from build123d import *

# Parameters (mm, degrees)
BOSS_EXTRUDE1_DEPTH       = 17.5
BOSS_EXTRUDE2_DEPTH       = 12.5
BOSS_EXTRUDE3_DEPTH       = 8
FILLET1_RADIUS            = 8
FILLET1_LENGTH            = 5
FILLET2_RADIUS            = 8
FILLET2_LENGTH            = 5
F_6_0MM_DOWEL_HOLE1_D     = 6
F_6_0MM_DOWEL_HOLE1_DEPTH = 21.06015
F_6_0MM_DOWEL_HOLE2_D     = 6
F_6_0MM_DOWEL_HOLE2_DEPTH = 12


with BuildPart() as part:
    # Sketch1 → Boss-Extrude1 (new, symmetric)
    with BuildSketch(Plane(origin=(0, 0, 0), x_dir=(0, 0, -1), z_dir=(1, 0, 0))):
        with BuildLine():
            Line((-7.858116823, -1.5), (-12.409673646, -1.5))
            ThreePointArc((-12.409673646, -1.5), (-8.291561976, -9.354143467), (0, -12.5))
            ThreePointArc((0, -12.5), (8.485281374, -16.014718626), (12, -24.5))
            Line((12, -24.5), (12, -33))
            Line((12, -33), (33, -33))
            Line((33, -33), (33, -3))
            Line((33, -3), (12.1346611, -3))
            ThreePointArc((12.1346611, -3), (2.254197856, 12.295063726), (-12.409673646, 1.5))
            Line((-12.409673646, 1.5), (-7.858116823, 1.5))
            ThreePointArc((-7.858116823, 1.5), (8, 0), (-7.858116823, -1.5))
        make_face()
    extrude(amount=BOSS_EXTRUDE1_DEPTH, both=True)

    # Sketch1<3> → Boss-Extrude2 (add, symmetric)
    with BuildSketch(Plane(origin=(0, 0, 0), x_dir=(0, 0, -1), z_dir=(1, 0, 0))):
        with BuildLine():
            ThreePointArc((-6, 10.9658561), (0, 12.5), (6, 10.9658561))
            Line((6, 10.9658561), (6, 25))
            Line((6, 25), (-6, 25))
            Line((-6, 25), (-6, 10.9658561))
        make_face()
    extrude(amount=BOSS_EXTRUDE2_DEPTH, both=True)

    # Sketch1<4> → Boss-Extrude3 (add, symmetric)
    with BuildSketch(Plane(origin=(0, 0, 0), x_dir=(0, 0, -1), z_dir=(1, 0, 0))):
        with BuildLine():
            ThreePointArc((-12.409673646, 1.5), (-11.810991842, 4.092734013), (-10.677078252, 6.5))
            Line((-10.677078252, 6.5), (-25, 6.5))
            Line((-25, 6.5), (-25, 1.5))
            Line((-25, 1.5), (-12.409673646, 1.5))
        make_face()
        with BuildLine():
            Line((-25, -6.5), (-10.677078252, -6.5))
            ThreePointArc((-10.677078252, -6.5), (-11.810991842, -4.092734013), (-12.409673646, -1.5))
            Line((-12.409673646, -1.5), (-25, -1.5))
            Line((-25, -1.5), (-25, -6.5))
        make_face()
    extrude(amount=BOSS_EXTRUDE3_DEPTH, both=True)

    # Fillet1: full round fillet: the end face becomes a half cylinder, R = half its width
    fillet1_face = Plane((0, 4, 25), x_dir=(0, 1, 0), z_dir=(0, 0, 1))  # on the end face: x along it, z out of the body
    fillet1_slab = fillet1_face.offset(-FILLET1_RADIUS / 2) * Box(FILLET1_LENGTH, 2 * FILLET1_RADIUS, FILLET1_RADIUS, mode=Mode.PRIVATE)  # the body's end, R deep
    fillet1_round = Plane((0, 4, 17), x_dir=(0, 0, 1), z_dir=(0, 1, 0)) * Cylinder(FILLET1_RADIUS, FILLET1_LENGTH, mode=Mode.PRIVATE)  # its axis R under the face
    add(fillet1_slab - fillet1_round, mode=Mode.SUBTRACT)

    # Fillet2: full round fillet: the end face becomes a half cylinder, R = half its width
    fillet2_face = Plane((0, -4, 25), x_dir=(0, -1, 0), z_dir=(0, 0, 1))  # on the end face: x along it, z out of the body
    fillet2_slab = fillet2_face.offset(-FILLET2_RADIUS / 2) * Box(FILLET2_LENGTH, 2 * FILLET2_RADIUS, FILLET2_RADIUS, mode=Mode.PRIVATE)  # the body's end, R deep
    fillet2_round = Plane((0, -4, 17), x_dir=(0, 0, 1), z_dir=(0, -1, 0)) * Cylinder(FILLET2_RADIUS, FILLET2_LENGTH, mode=Mode.PRIVATE)  # its axis R under the face
    add(fillet2_slab - fillet2_round, mode=Mode.SUBTRACT)

    # Ø6.0mm Dowel Hole1
    with Locations(Plane(origin=(0, 6.5, 17), x_dir=(0, 0, 1), z_dir=(0, 1, 0))):
        with Locations((0, 0)):
            Hole(F_6_0MM_DOWEL_HOLE1_D / 2, depth=F_6_0MM_DOWEL_HOLE1_DEPTH)

    # Ø6.0mm Dowel Hole2
    with Locations(Plane.ZX.offset(25)):
        with Locations((0, 0)):
            Hole(F_6_0MM_DOWEL_HOLE2_D / 2, depth=F_6_0MM_DOWEL_HOLE2_DEPTH)


solid = part.part
Read the model definition and answer for the solid it produces. Units are mm, in the model's axes. A direction names the side the tool comes from. Coordinates: 2 decimals unless noted, no trailing zeros. Loops run counter-clockwise (first coordinate to the right, second up) from the corner with the lowest first, then second, coordinate; pieces in that order, holes last.
Q1. The part is cut by section C-C on x = 15. Write down the section's boundary in (y, z), and give its area (3 significant figures).
Q2. The part is cut by section A-A on x = 0. Give the number of separate pieces and of enclosed holes in the cut face, and give its area (3 significant figures).
Q3. Which of the six approach directions +Z, -Z, +X, -X, +Y, -Y give full straight-line access (tool end or side, diameter ignored) to faces 1 (the face through (-4, 6.5, 18)), 2 (the face through (0, -1.5, 12)), 3 (the face through (0, 18, -6))?
Q4. Each of these flat-tipped pins is pushed along its axis until it touches: pin 1 Ø5 at (y, z) = (-15.5, -2) entering from +X; pin 2 Ø4.5 at (x, z) = (3.5, 21.5) entering from +Y; pin 3 Ø5 at (x, z) = (0, 0) entering from +Y; pin 4 Ø7 at (x, y) = (-5, 20.5) entering from -Z. Where does it stop, or does it pass through?
Q5. The mould has two halves that part along X. Classify faces 4 (the face through (0, 4, 25)), 5 (the face through (0, 18, 6)), 6 (the face through (0, -4, 20)): +X half, -X half, draft (parallel to the pull), parting line (faces both ways), or undercut.
Q6. Consider probe 1 along Y at (x, z) = (-2, 20.5); probe 2 along X at (y, z) = (18, 0); probe 3 along X at (y, z) = (-4, 17). Determine where each line is inside the solid, lowest interval first.
Q7. The part is cut by section B-B on y = 16.5. Write down the section's boundary in (x, z).
Q8. The part is cut by section D-D on z = 18.5. Write down the section's boundary in (x, y), and give its area (3 significant figures).
Results below:
1. outline: (-33, -33) - (-3, -33) - (-3, -12.13) arc R12.5 ccw (long way) to (1.5, 12.41) - (1.5, 7.86) arc R8 cw (long way) to (-1.5, 7.86) - (-1.5, 12.41) arc R12.5 ccw to (-12.5, 0) arc R12 cw to (-24.5, -12) - (-33, -12) - close
1. area: 966 mm2
2. separate pieces: 3
2. enclosed holes: 0
2. area: 1,120 mm2
3. face 1: +Z, +X, -X, +Y
3. face 2: +Z, +X, -X
3. face 3: -Z, +X, -X, +Y
4. pin 1: passes through
4. pin 2: stops at y = 6.5
4. pin 3: stops at y = 13
4. pin 4: stops at z = -6
5. face 4: parting line
5. face 5: draft
5. face 6: undercut
6. probe 1: y = -6.5 to -1.5, 1.5 to 6.5
6. probe 2: x = -12.5 to -3, 3 to 12.5
6. probe 3: x = -8 to -3, 3 to 8
7. outline: (-12.5, -6) - (12.5, -6) - (12.5, 6) - (-12.5, 6) - close; hole circle Ø6 at (0, 0)
8. outline: (-7.86, -6.5) - (-2.6, -6.5) - (-2.6, -1.5) - (-7.86, -1.5) - close; (-7.86, 1.5) - (-2.6, 1.5) - (-2.6, 6.5) - (-7.86, 6.5) - close; (2.6, -6.5) - (7.86, -6.5) - (7.86, -1.5) - (2.6, -1.5) - close; (2.6, 1.5) - (7.86, 1.5) - (7.86, 6.5) - (2.6, 6.5) - close
8. area: 105 mm2
